For this review, take the finished solid that the model builds, in its own axes (mm). A direction names the side the tool comes from. Coordinates: 2 decimals unless noted, no trailing zeros. Loops run counter-clockwise (first coordinate to the right, second up) from the corner with the lowest first, then second, coordinate; pieces in that order, holes last.
1. Machinability: for faces 4 (the face through (19, 0, 10)), 5 (the face through (27.84, 3.45, -21.71)), 6 (the face through (10.382, 13.944, -19.961)), which of the approach directions +Z, -Z, +X, -X, +Y, -Y give a long, thin tool a straight path to every point of the face, cutting with its end or side? Answer none if there is none.
2. Take a section at C-C, the plane x = 0. Count the separate pieces of the cut face and the enclosed holes in it, then the cut area to 3 significant figures.
3. Take a section at A-A, the plane z = 0. State the section outline as (x, y) points.
4. Take a section at B-B, the plane y = 14.25. State the section outline as (x, z) points.
5. To check wall thickness, follow probe 1 along X at (y, z) = (5, 23); probe 2 along Z at (x, y) = (35, 7.75); probe 3 along Z at (x, y) = (35, 3.5). State the ranges of each line that lie inside material, in increasing order.
6. Mouldability with a two-part tool opening along Z and no side actions: class faces 1 (the face through (-4.036, 14.19, -30.736)), 2 (the face through (-27.84, 3.45, 21.71)), 3 (the face through (-13, 10, 30)) as pulls with the +Z half, pulls with the -Z half, needs draft (parallel to the pull), parting line crosses it, or undercut.
7. Clearance check with flat-ended pins moving along their axes: P1, Ø1.5, axis at x = 35, y = 5, coming from the -Z side; P2, Ø10, axis at x = 16.5, y = 9, coming from the -Z side; P3, Ø3, axis at y = 2, z = -11.5, coming from the +X side; P4, Ø5.5, axis at x = 32.48, z = -18.75, coming from the -Y side. State where each tip first meets the part, or that it passes through.
Autodesk Inventor part; units mm, degrees
ref_plane "YZ Plane" through (0, 0, 0) normal (1, 0, 0) x (0, 1, 0)
ref_plane "XZ Plane" through (0, 0, 0) normal (0, 1, 0) x (-1, 0, 0)
ref_plane "XY Plane" through (0, 0, 0) normal (0, 0, 1) x (1, 0, 0)
sketch "Эскиз1" plane through (0, 0, 0) normal (0, 0, 1) x (1, 0, 0)
  line L0 (0, 8.5) -> (0, 0)
  line L1 (0, 0) -> (31, 0)
  line L2 (31, 0) -> (31, 18)
  line L3 (31, 18) -> (22.5, 18)
  line L4 (22.5, 18) -> (22.5, 8.5)
  line L5 (22.5, 8.5) -> (0, 8.5)
  dimension "d0" = 18
  dimension "d3" = 31
  dimension "d28" = 22.5
revolve "Вращение1" add sketch "Эскиз1" angle 360 about axis through (0, 8.5, 0) along (0, -1, 0)
sketch "Эскиз2" plane through (0, 0, 0) normal (1, 0, 0) x (0, 1, 0)
  line L0 (0, 31) -> (0, -31)
  line L1 (18, 31) -> (0, 31)
  line L2 (18, 31) -> (0, 31)
  line L3 (0, 0) -> (0, 45)
  line L4 (0, 45) -> (10, 45)
  line L5 (10, 45) -> (10, 0)
  line L6 (10, 0) -> (0, 0)
  line L7 (-3, 0) -> (18, 0)
  dimension "d5" = 10
  dimension "d6" = 45
revolve "Вращение2" add sketch "Эскиз2" angle 360 about axis through (0, -10, 0) along (0, 1, 0)
sketch "Эскиз3" plane through (0, 0, 0) normal (0, -1, 0) x (1, 0, 0)
  line L0 (0, -63) -> (0, 63)
  line L1 (-63, 0) -> (63, 0)
  circle A0 centre (0, 0) radius 37.5 construction
  circle A1 centre (0, 37.5) radius 5.5
  point P0 (0, 0)
  dimension "d8" = 75
  dimension "d9" = 11
hole "Отверстие1" at (0, 0, 37.5) direction (0, 1, 0) diameter 6.2 depth 15 tip angle 118 counterbore diameter 11 counterbore depth 6.8
pattern_circular "Круговой массив1" count 6 over 360 about axis through (0, -10, 0) along (0, 1, 0) of "Отверстие1"
fillet "Сопряжение1" radius 1.3 1 edges at (-31, 10, 0)
chamfer "Фаска1" distance 1 angle 45 1 edges at (0, 0, -45)
sketch "Эскиз5" plane through (0, 0, 0) normal (0, -1, 0) x (1, 0, 0)
  line L0 (0, 63) -> (0, -63)
  line L1 (-63, 0) -> (63, 0)
  circle A0 centre (0, 0) radius 20
  point P0 (0, 0)
  dimension "d25" = 40
extrude "Выдавливание1" cut sketch "Эскиз5" against normal blind 15
chamfer "Фаска2" distance 1 angle 45 1 edges at (-20, 0, 0)
chamfer "Фаска3" distance 1 angle 45 1 edges at (-31, 18, 0)
properties part number "Крышка маленькая_под манж_01"
Results list:
1. face 4: +Z, -Z, +X, -X, -Y
1. face 5: -Y
1. face 6: +Y
2. separate pieces: 4
2. enclosed holes: 0
2. area: 444 mm2
3. outline: (-45, 1) - (-44, 0) - (-21, 0) - (-20, 1) - (-20, 10) - (-22.5, 10) - (-22.5, 18) - (-30, 18) - (-31, 17) - (-31, 11.3) arc R1.3 cw to (-32.3, 10) - (-45, 10) - close; (20, 1) - (21, 0) - (44, 0) - (45, 1) - (45, 10) - (32.3, 10) arc R1.3 cw to (31, 11.3) - (31, 17) - (30, 18) - (22.5, 18) - (22.5, 10) - (20, 10) - close
4. outline: circle Ø62 at (0, 0); hole circle Ø45 at (0, 0)
5. probe 1: x = -38.68 to -35.97, -28.98 to 28.98, 35.97 to 38.68
5. probe 2: z = -28.28 to -20.55, -16.95 to 16.95, 20.55 to 28.28
5. probe 3: z = -28.28 to -23.64, -13.86 to 13.86, 23.64 to 28.28
6. face 1: parting line crosses it
6. face 2: undercut
6. face 3: needs draft
7. P1: stops at z = -29.19
7. P2: stops at z = -43.51
7. P3: stops at x = 43.87
7. P4: passes through
